from build123d import *

# Parameters (mm, degrees)
SKETCH1_W           = 69.85
SKETCH1_H           = 6.35
BOSS_EXTRUDE1_DEPTH = 120.65
CUT_EXTRUDE1_DEPTH  = 140.555607197


with BuildPart() as part:
    # Sketch1 → Boss-Extrude1 (new body)
    with BuildSketch(Plane.XY):
        with Locations((34.925, 3.175)):
            Rectangle(SKETCH1_W, SKETCH1_H)
    extrude(amount=BOSS_EXTRUDE1_DEPTH)

    # Sketch2 → Cut-Extrude1 (cut, through all)
    with BuildSketch(Plane(origin=(0, 6.35, 0), x_dir=(1, 0, 0), z_dir=(0, 1, 0))):
        Polygon((35.923749516, 0), (35.923749516, -37.802999389), (69.85, -55.962276793), (69.85, 0), align=None)
    extrude(amount=-CUT_EXTRUDE1_DEPTH, mode=Mode.SUBTRACT)


solid = part.part
Could you check a few things on this model? Use its own coordinates, in mm. A direction names the side the tool comes from. Coordinates: 2 decimals unless noted, no trailing zeros. Order: outer loops, then holes, each group sorted by start corner. A loop starts at its lowest first (then second) coordinate and runs counter-clockwise, first axis right, second up. Notation, with made-up numbers: (76, 24.5) -> (111, 24.5) arc R9 cw to (111, 39.5) -> close; hole circle Ø8 at (-23, 26.5). An arc over 180 degrees is marked (long way). One line per item, written item: value. Start each with the question number.
1) If I drill on L1, parallel to X at y = 6, z = 29.5; L2, parallel to Z at x = 46, y = 2.5; L3, parallel to Z at x = 54.5, y = 4.5, over which ranges is the centre line in solid material (lowest first)? Write a range as [from, to].
2) Imagine slicing it at B-B on z = 15.5. List the corners of the cut face in (x, y) for me, plus the area to 3 significant figures.
3) I'm going to push flat-ended pins straight in: pin 1 (1 mm diameter, centred on y = 1, z = 22, fed in from +X); pin 2 (2 mm diameter, centred on y = 5, z = 50, fed in from +X). Where does each tip first touch, or does it pass through?
4) Imagine slicing it at C-C on x = 44. List the corners of the cut face in (y, z) for me.
5) Which directions (+Z, -Z, +X, -X, +Y, -Y) give clear straight access to the entire face, cutting with the end or side of a thin tool? Please do faces 1 (the flat face through (18, 3, 0)), 2 (the flat face through (35.924, 3, 19)).
6) Imagine slicing it at A-A on y = 1. List the corners of the cut face in (x, z) for me, plus the area to 3 significant figures.
Answer list:
1. L1: x = [0, 35.92]
1. L2: z = [43.2, 120.65]
1. L3: z = [47.75, 120.65]
2. outline: (0, 0) -> (35.92, 0) -> (35.92, 6.35) -> (0, 6.35) -> close
2. area: 228 mm2
3. pin 1: stops at x = 35.92
3. pin 2: stops at x = 60.58
4. outline: (0, 42.13) -> (6.35, 42.13) -> (6.35, 120.65) -> (0, 120.65) -> close
5. face 1: -Z, +X, -X, +Y, -Y
5. face 2: -Z, +X, +Y, -Y
6. outline: (0, 0) -> (35.92, 0) -> (35.92, 37.8) -> (69.85, 55.96) -> (69.85, 120.65) -> (0, 120.65) -> close
6. area: 6,840 mm2
